Geometry: see drawing. Coordinates: mm, zero at the bounding-box minimum. Coordinates: 2 decimals unless noted, no trailing zeros. Loops run counter-clockwise (first coordinate to the right, second up) from the corner with the lowest first, then second, coordinate; pieces in that order, holes last. Notation, with made-up numbers: (-20.75, -14) - (-11.75, -14) arc R7 ccw to (-11.75, -6) - close; hole circle Ø1 at (-13.75, 23.25). An arc over 180 degrees is marked (long way). Answer in a Markdown table with one row per item.
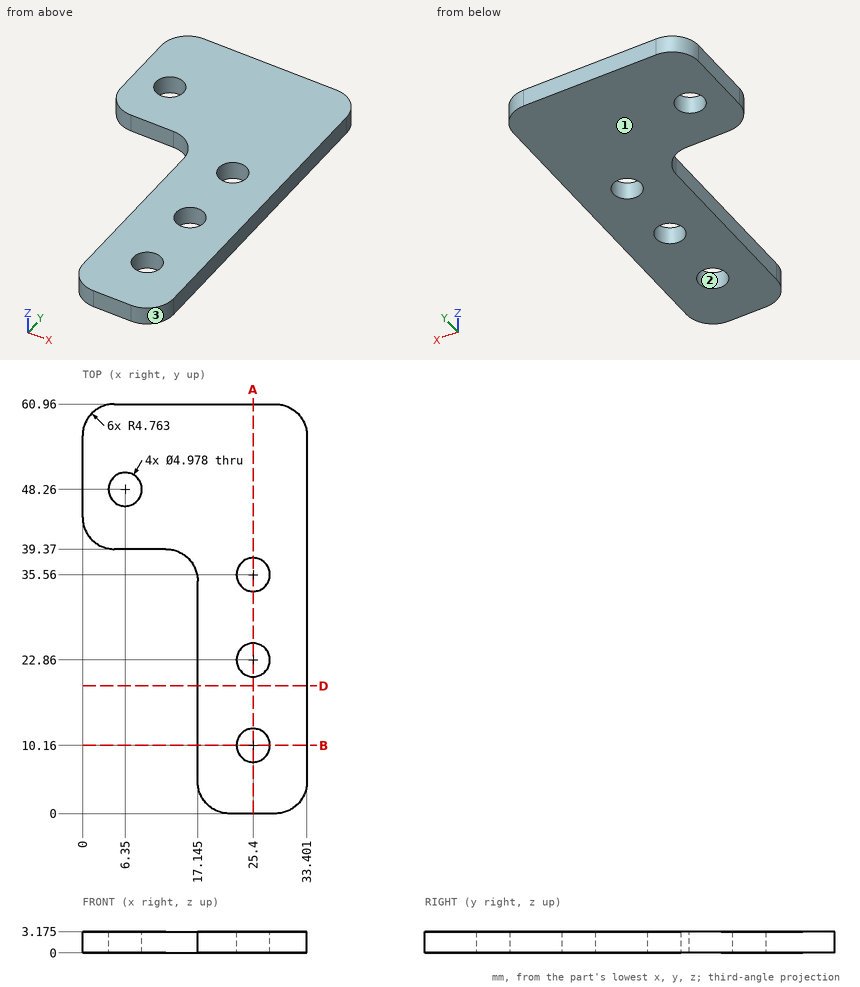
(1) Cut plane A-A on x = 25.4. State how many separate pieces and enclosed holes the cut face has, then the cut area to 3 significant figures.
Verdict:
| item | result |
|---|---|
| separate pieces | 4 |
| enclosed holes | 0 |
| area | 146 mm² |
(2) Cut plane B-B on y = 10.16. Output: boundary loops of the cut face in (x, z) (1 decimal), then the cut area to 3 significant figures.
Verdict:
| item | result |
|---|---|
| outline | (17.1, 0) - (22.9, 0) - (22.9, 3.2) - (17.1, 3.2) - close; (27.9, 0) - (33.4, 0) - (33.4, 3.2) - (27.9, 3.2) - close |
| area | 35.8 mm² |
(3) Cut plane D-D on y = 19. Output: boundary loops of the cut face in (x, z) (1 decimal).
Verdict:
| item | result |
|---|---|
| outline | (17.1, 0) - (33.4, 0) - (33.4, 3.2) - (17.1, 3.2) - close |
(4) Pull-direction query (Y, two-part tool) for the marked faces 1, 2 and 3; classes: pulls with the +Y half, pulls with the -Y half, needs draft (parallel to the pull), parting line crosses it, or undercut.
Verdict:
| item | result |
|---|---|
| face 1 | needs draft |
| face 2 | undercut |
| face 3 | pulls with the -Y half |
(5) Ray query, probe 1 along Y at (x, z) = (25.4, 1.2); probe 2 along X at (y, z) = (48.5, 1.25); probe 3 along Y at (x, z) = (6.35, 1). Return the intervals inside material, ascending.
Verdict:
| item | result |
|---|---|
| probe 1 | y = 0 to 7.67, 12.65 to 20.37, 25.35 to 33.07, 38.05 to 60.96 |
| probe 2 | x = 0 to 3.87, 8.83 to 33.4 |
| probe 3 | y = 39.37 to 45.77, 50.75 to 60.96 |
